Source: CAD feature listing. Evaluate the final solid. Frame: model axes, mm. A direction names the side the tool comes from. Give positions to 0.01 mm unless a question says otherwise; leave off trailing zeros. Loops run counter-clockwise (first coordinate to the right, second up) from the corner with the lowest first, then second, coordinate; pieces in that order, holes last.
from build123d import *

# Parameters (mm, degrees)
F0_W     = 200
F0_H     = 50
F1_DEPTH = 75
F2_W     = 127.414032
F2_H     = 182.310182
F3_DEPTH = 20
F5_W     = 126.305566
F5_H     = 177.75355
F6_DEPTH = 27
F4_W     = 20
F4_H     = 9
F7_DEPTH = 25
F9_DEPTH = 160


with BuildPart() as f1:
    # F0 (on Right) → F1 (new body, symmetric)
    with BuildSketch(Plane.YZ):
        with Locations((100, 25)):
            Rectangle(F0_W, F0_H)
    extrude(amount=F1_DEPTH, both=True)

    # F2 (on face) → F3 (cut)
    with BuildSketch(Plane.XY.offset(50)):
        with Locations((0, 100)):
            Rectangle(F2_W, F2_H)
    extrude(amount=-F3_DEPTH, mode=Mode.SUBTRACT)

    # F5 (on face) → F6 (cut)
    with BuildSketch(Plane(origin=(0, 0, 0), x_dir=(1, 0, 0), z_dir=(0, 0, -1))):
        with Locations((0, -100)):
            Rectangle(F5_W, F5_H)
    extrude(amount=-F6_DEPTH, mode=Mode.SUBTRACT)

    # F4 (on face) → F7 (cut)
    with BuildSketch(Plane.XZ):
        with Locations((45, 4.5)):
            Rectangle(F4_W, F4_H)
        with Locations((-44.462749, 4.5)):
            Rectangle(F4_W, F4_H)
    extrude(amount=-F7_DEPTH, mode=Mode.SUBTRACT)

    # F8 (on face) → F9 (cut)
    with BuildSketch(Plane.YZ.offset(75)):
        with BuildLine():
            Line((60, 14), (60, 0))
            Line((60, 0), (110, 0))
            Line((110, 0), (110, 14))
            ThreePointArc((110, 14), (107.071068, 21.071068), (100, 24))
            Line((100, 24), (70, 24))
            ThreePointArc((70, 24), (62.928932, 21.071068), (60, 14))
        make_face()
    extrude(amount=-F9_DEPTH, mode=Mode.SUBTRACT)


solid = f1.part
1) Reachability of faces 1 (the cylindrical face through (69.16, 107.15, 20.99)), 2 (the flat face through (-1, 11.123, 13)), 3 (the flat face through (67, 23, 0)), 4 (the flat face through (-45, 5, 9)), 5 (the flat face through (-1, 191.155, 40)) from +Z, -Z, +X, -X, +Y, -Y: full face, straight path, thin tool, end or side. Return the list, or none.
Checks:
face 1: -Z, +X, -X
face 2: -Z
face 3: -Z, +X, -X, +Y, -Y
face 4: -Z, -Y
face 5: +Z
2) Ray query, probe 1 along Y at (x, z) = (16, 40); probe 2 along X at (y, z) = (154.5, 40.5); probe 3 along Y at (x, z) = (-22, 3). Return the intervals inside material, ascending.
Checks:
probe 1: y = 0 to 8.84, 191.16 to 200
probe 2: x = -75 to -63.71, 63.71 to 75
probe 3: y = 0 to 11.12, 188.88 to 200
3) Cut plane A-A (x = -48). Return loops of the section in (y, z), and give its area (3 significant figures).
Checks:
outline: (0, 9) - (11.12, 9) - (11.12, 27) - (188.88, 27) - (188.88, 0) - (200, 0) - (200, 50) - (191.16, 50) - (191.16, 30) - (8.84, 30) - (8.84, 50) - (0, 50) - close
area: 1,450 mm2
4) Cut plane D-D (z = 17). Return loops of the section in (x, y), and give its area (3 significant figures).
Checks:
outline: (-75, 0) - (75, 0) - (75, 60.46) - (63.15, 60.46) - (63.15, 11.12) - (-63.15, 11.12) - (-63.15, 60.46) - (-75, 60.46) - close; (-75, 109.54) - (-63.15, 109.54) - (-63.15, 188.88) - (63.15, 188.88) - (63.15, 109.54) - (75, 109.54) - (75, 200) - (-75, 200) - close
area: 6,390 mm2
5) Cut plane C-C (y = 94). Return loops of the section in (x, z).
Checks:
outline: (-75, 24) - (-63.15, 24) - (-63.15, 27) - (63.15, 27) - (63.15, 24) - (75, 24) - (75, 50) - (63.71, 50) - (63.71, 30) - (-63.71, 30) - (-63.71, 50) - (-75, 50) - close
6) Cut plane B-B (z = 46). Return loops of the section in (x, y), and give its area (3 significant figures).
Checks:
outline: (-75, 0) - (75, 0) - (75, 200) - (-75, 200) - close; hole (-63.71, 8.84) - (63.71, 8.84) - (63.71, 191.16) - (-63.71, 191.16) - close
area: 6,770 mm2
7) Pull-direction query (Y, two-part tool) for faces 6 (the flat face through (63.707, 99, 40)), 7 (the flat face through (45, 5, 9)), 8 (the flat face through (63.153, 121, 13)); classes: released by +Y, released by -Y, zero draft, split by the parting line, or undercut.
Checks:
face 6: undercut
face 7: zero draft
face 8: undercut
8) Contact query for flat-ended pins moving along their axis: P1, Ø1, axis at x = 9.5, y = 165, coming from the +Z side; P2, Ø8, axis at x = 28, y = 161, coming from the -Z side; P3, Ø3.5, axis at x = 67, y = 81, coming from the -Z side. Output: stop coordinate, or through.
Checks:
P1: stops at z = 30
P2: stops at z = 27
P3: stops at z = 24
